from build123d import *

# Parameters (mm, degrees)
SKETCH1_W                                        = 101.6
SKETCH1_H                                        = 50.8
BOSS_EXTRUDE1_DEPTH                              = 25.4
CBORE_FOR_1_4_SOCKET_HEAD_CAP_SCREW1_D           = 6.7564
CBORE_FOR_1_4_SOCKET_HEAD_CAP_SCREW1_CBORE_D     = 11.1125
CBORE_FOR_1_4_SOCKET_HEAD_CAP_SCREW1_CBORE_DEPTH = 6.35
LPATTERN1_COUNT                                  = 2
LPATTERN1_PITCH                                  = 25.4
LPATTERN1_COUNT_DIR2                             = 4
LPATTERN1_PITCH_DIR2                             = 25.4
F_1_4_20_TAPPED_HOLE1_D                          = 5.1054
LPATTERN2_COUNT                                  = 2
LPATTERN2_PITCH                                  = 25.4
LPATTERN2_COUNT_DIR2                             = 3
LPATTERN2_PITCH_DIR2                             = 25.4


with BuildPart() as part:
    # Sketch1 → Boss-Extrude1 (new body)
    with BuildSketch(Plane(origin=(0, 0, 0), x_dir=(1, 0, 0), z_dir=(0, 1, 0))):
        with Locations((50.8, 25.4)):
            Rectangle(SKETCH1_W, SKETCH1_H)
    extrude(amount=BOSS_EXTRUDE1_DEPTH)

    # CBORE for 1/4 Socket Head Cap Screw1 (through all)
    with Locations(Plane(origin=(0, 25.4, 0), x_dir=(-1, 0, 0), z_dir=(0, 1, 0))):
        with Locations((-12.7, -12.7)):
            cbore_for_1_4_socket_head_cap_screw1 = CounterBoreHole(CBORE_FOR_1_4_SOCKET_HEAD_CAP_SCREW1_D / 2, CBORE_FOR_1_4_SOCKET_HEAD_CAP_SCREW1_CBORE_D / 2, CBORE_FOR_1_4_SOCKET_HEAD_CAP_SCREW1_CBORE_DEPTH)

    # LPattern1: CBORE for 1_4 Socket Head Cap Screw1 2 × 4
    with Locations(*[(j * LPATTERN1_PITCH_DIR2, 0, -i * LPATTERN1_PITCH) for i in range(LPATTERN1_COUNT) for j in range(LPATTERN1_COUNT_DIR2) if (i, j) != (0, 0)]):
        add(cbore_for_1_4_socket_head_cap_screw1, mode=Mode.SUBTRACT)

    # 1/4-20 Tapped Hole1 (through all)
    with Locations(Plane(origin=(0, 25.4, 0), x_dir=(-1, 0, 0), z_dir=(0, 1, 0))):
        with Locations((-25.4, -38.1)):
            f_1_4_20_tapped_hole1 = Hole(F_1_4_20_TAPPED_HOLE1_D / 2)

    # LPattern2: 1_4-20 Tapped Hole1 2 × 3
    with Locations(*[(j * LPATTERN2_PITCH_DIR2, 0, i * LPATTERN2_PITCH) for i in range(LPATTERN2_COUNT) for j in range(LPATTERN2_COUNT_DIR2) if (i, j) != (0, 0)]):
        add(f_1_4_20_tapped_hole1, mode=Mode.SUBTRACT)


solid = part.part
Could you check a few things on this model? Use its own coordinates, in mm. A direction names the side the tool comes from. Coordinates: 2 decimals unless noted, no trailing zeros. Order: outer loops, then holes, each group sorted by start corner. A loop starts at its lowest first (then second) coordinate and runs counter-clockwise, first axis right, second up. Notation, with made-up numbers: (52, -3) -> (86, -3) arc R13 cw to (86, 11) -> close; hole circle Ø10 at (55.25, -36.5). An arc over 180 degrees is marked (long way). One line per item, written item: value. Start each with the question number.
1) We'd pull the mould along X, two halves only. Please class faces 1 (the flat face through (38.2, 19.05, -16.3)), 2 (the flat face through (50, 13, -50.8)): +X half, -X half, draft (parallel to the pull), parting line (faces both ways), or undercut.
2) I'm going to push a flat-ended pin straight in: pin 1 (9 mm diameter, centred on x = 88.9, z = -38.1, fed in from +Y). Where does the tip first touch, or does it pass through?
3) Imagine slicing it at A-A on x = 76.2. List the corners of the cut face in (y, z) for me, plus the area to 3 significant figures.
4) Imagine slicing it at D-D on x = 63.5. List the corners of the cut face in (y, z) for me, plus the area to 3 significant figures.
5) Imagine slicing it at B-B on y = 14.25. Count the separate pieces of the cut face and the enclosed holes in it, plus the area to 3 significant figures.
6) If I drill on L1, parallel to Z at x = 84.5, y = 19.75; L2, parallel to Z at x = 25.4, y = 7.25; L3, parallel to Y at x = 13, z = -8.5, over which ranges is the centre line in solid material (lowest first)? Write a range as [from, to].
7) Which directions (+Z, -Z, +X, -X, +Y, -Y) give clear straight access to the entire face, cutting with the end or side of a thin tool? Please do faces 3 (the cylindrical face through (62.77, 9.39, -16)), 4 (the flat face through (89, 19.05, -42)).
Answer list:
1. face 1: undercut
1. face 2: draft
2. pin 1: stops at y = 19.05
3. outline: (0, -50.8) -> (25.4, -50.8) -> (25.4, -40.65) -> (0, -40.65) -> close; (0, -35.55) -> (25.4, -35.55) -> (25.4, -15.25) -> (0, -15.25) -> close; (0, -10.15) -> (25.4, -10.15) -> (25.4, 0) -> (0, 0) -> close
3. area: 1,030 mm2
4. outline: (0, -50.8) -> (25.4, -50.8) -> (25.4, -43.66) -> (19.05, -43.66) -> (19.05, -41.48) -> (0, -41.48) -> close; (0, -34.72) -> (19.05, -34.72) -> (19.05, -32.54) -> (25.4, -32.54) -> (25.4, -18.26) -> (19.05, -18.26) -> (19.05, -16.08) -> (0, -16.08) -> close; (0, -9.32) -> (19.05, -9.32) -> (19.05, -7.14) -> (25.4, -7.14) -> (25.4, 0) -> (0, 0) -> close
4. area: 892 mm2
5. separate pieces: 1
5. enclosed holes: 14
5. area: 4,750 mm2
6. L1: z = [-50.8, -41.49], [-34.71, -16.09], [-9.31, 0]
6. L2: z = [-50.8, -40.65], [-35.55, -15.25], [-10.15, 0]
6. L3: y = [0, 19.05]
7. face 3: +Y, -Y
7. face 4: +Y
